Could you check a few things on this model? Use its own coordinates, in mm. Face numbers are marked on the shaded views. A direction names the side the tool comes from. Coordinates: 2 decimals unless noted, no trailing zeros. Order: outer loops, then holes, each group sorted by start corner. A loop starts at its lowest first (then second) coordinate and runs counter-clockwise, first axis right, second up.
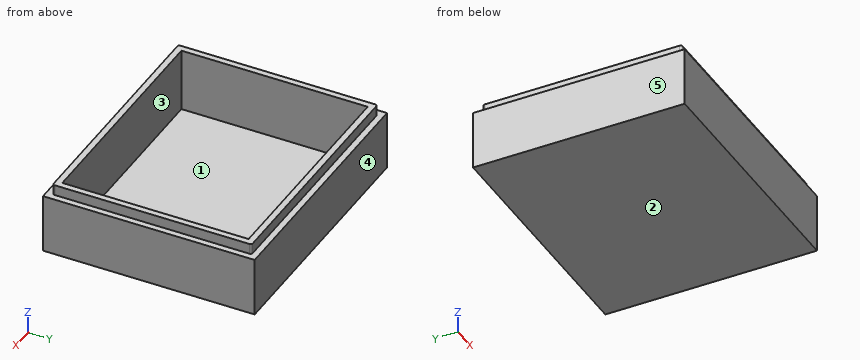
```python
from build123d import *

# Parameters (mm, degrees)
CROQUIS1_W              = 120
CROQUIS1_H              = 100
SALIENTE_EXTRUIR1_DEPTH = 3
CROQUIS3_W              = 120
CROQUIS3_H              = 100
CROQUIS3_W_2            = 114
CROQUIS3_H_2            = 94
SALIENTE_EXTRUIR2_DEPTH = 25
CROQUIS4_W              = 114
CROQUIS4_H              = 94
CROQUIS4_W_2            = 108
CROQUIS4_H_2            = 88
SALIENTE_EXTRUIR3_DEPTH = 30
REDONDEO1_R             = 1


with BuildPart() as part:
    # Croquis1 → Saliente-Extruir1 (new body)
    with BuildSketch(Plane.XY):
        with Locations((60, 50)):
            Rectangle(CROQUIS1_W, CROQUIS1_H)
    extrude(amount=SALIENTE_EXTRUIR1_DEPTH)

    # Croquis3 → Saliente-Extruir2 (add)
    with BuildSketch(Plane.XY.offset(3)):
        with Locations((60, 50)):
            Rectangle(CROQUIS3_W, CROQUIS3_H)
        with Locations((60, 50)):
            Rectangle(CROQUIS3_W_2, CROQUIS3_H_2, mode=Mode.SUBTRACT)
    extrude(amount=SALIENTE_EXTRUIR2_DEPTH)

    # Croquis4 → Saliente-Extruir3 (add)
    with BuildSketch(Plane.XY.offset(3)):
        with Locations((60, 50)):
            Rectangle(CROQUIS4_W, CROQUIS4_H)
        with Locations((60, 50)):
            Rectangle(CROQUIS4_W_2, CROQUIS4_H_2, mode=Mode.SUBTRACT)
    extrude(amount=SALIENTE_EXTRUIR3_DEPTH)

    # Redondeo1
    redondeo1_edges = [part.edges().sort_by_distance(p)[0] for p in [
        (3, 97, 30.5),
        (3, 3, 30.5),
        (117, 3, 30.5),
        (117, 97, 30.5),
    ]]
    fillet(redondeo1_edges, radius=REDONDEO1_R)


solid = part.part
```
Item 1: Suppose I cut it at A-A (z = 10.5). List the corners of the cut face in (x, y) for me, and give its area (3 significant figures).
Item 2: I need wall thicknesses on line 1 (X direction, y = 15.5, z = 4); line 2 (Y direction, x = 85, z = 7); line 3 (X direction, y = 26, z = 29.5). Which ranges of each line are inside material? Lowest first, please.
Item 3: Which directions (+Z, -Z, +X, -X, +Y, -Y) give clear straight access to the entire face, cutting with the end or side of a thin tool? Please do the marked faces 1 and 2.
Item 4: Thinking about a two-plate mould opening in Y: for the marked faces 3, 4 and 5, which applies, +Y half, -Y half, draft (parallel to the pull), parting line (faces both ways), or undercut?
Item 5: For pin 1 Ø5.5 at (y, z) = (60, 30.5) entering from +X; pin 2 Ø12 at (x, y) = (28, 51) entering from +Z; pin 3 Ø1.5 at (x, z) = (36, 30.5) entering from -Y; pin 4 Ø2.5 at (y, z) = (34, 30.5) entering from -X, each with a flat end and sliding along its axis, tell me the tip position at first contact or that it passes through.
Item 6: Suppose I cut it at B-B (x = 32). List the corners of the cut face in (y, z) for me.
Item 7: Suppose I cut it at C-C (y = 90.5). List the corners of the cut face in (x, z) for me.
Geometry results:
1. outline: (0, 0) - (120, 0) - (120, 100) - (0, 100) - close; hole (6, 6) - (114, 6) - (114, 94) - (6, 94) - close
1. area: 2,500 mm2
2. line 1: x = 0 to 6, 114 to 120
2. line 2: y = 0 to 6, 94 to 100
2. line 3: x = 3 to 6, 114 to 117
3. face 1: +Z
3. face 2: -Z, +X, -X, +Y, -Y
4. face 3: undercut
4. face 4: +Y half
4. face 5: draft
5. pin 1: stops at x = 120
5. pin 2: stops at z = 3
5. pin 3: stops at y = 3
5. pin 4: stops at x = 3
6. outline: (0, 0) - (100, 0) - (100, 28) - (97, 28) - (97, 33) - (94, 33) - (94, 3) - (6, 3) - (6, 33) - (3, 33) - (3, 28) - (0, 28) - close
7. outline: (0, 0) - (120, 0) - (120, 28) - (117, 28) - (117, 33) - (114, 33) - (114, 3) - (6, 3) - (6, 33) - (3, 33) - (3, 28) - (0, 28) - close
